Work out the finished part from the listing and answer in its coordinate system (mm). A direction names the side the tool comes from. Round coordinates to 2 decimals unless told otherwise and drop trailing zeros. Order: outer loops, then holes, each group sorted by start corner. A loop starts at its lowest first (then second) coordinate and runs counter-clockwise, first axis right, second up. Notation, with made-up numbers: (3, 3.5) - (8, 3.5) arc R31 cw to (8, 27.5) - close; hole circle Ø8 at (70, 70.25). An arc over 180 degrees is marked (long way). One line per question, with ' | ' between items. Start each with the question number.
from build123d import *

# Parameters (mm, degrees)
F1_DEPTH = 1285
F2_W     = 650
F2_H     = 250
F3_DEPTH = 650


with BuildPart() as f1:
    # F0 (on Front) → F1 (new body)
    with BuildSketch(Plane.XZ):
        Polygon((-600, 0), (0, 0), (600, 0), (600, 550), (550, 600), (-550, 600), (-600, 550), align=None)
    extrude(amount=F1_DEPTH)

    # F2 (on face) → F3 (cut)
    with BuildSketch(Plane.XZ.offset(1285)):
        with Locations((0, 125)):
            Rectangle(F2_W, F2_H)
    extrude(amount=-F3_DEPTH, mode=Mode.SUBTRACT)


solid = f1.part
1) Determine the mould class of faces 1 (the flat face through (-325, -965, 123)), 2 (the flat face through (-8, -491, 0)), 3 (the flat face through (-5, -965, 250)), 4 (the flat face through (-600, -634, 279)) for opening direction X: released by +X, released by -X, zero draft, split by the parting line, or undercut.
2) Section C-C on z = 46.5 is taken. Give the vertices of the cut face in (x, y).
3) For faces 5 (the flat face through (-575, -634, 575)), 6 (the flat face through (-5, -635, 127)), determine the directions among +Z, -Z, +X, -X, +Y, -Y from which every point of the face is accessible in a straight line to the end or side of a thin tool.
4) Section A-A on y = -795 is taken. Give the vertices of the cut face in (x, z), and give its area (3 significant figures).
5) Straight lines are drawn through the part: line 1 (Z direction, x = -2.5, y = -1100); line 2 (Y direction, x = -83, z = 40); line 3 (X direction, y = -958, z = 229). For each, find the intervals that lie inside material, in ascending order.
6) A flat-ended cylindrical pin translates along its axis: pin 1 (4 mm diameter, centred on x = 149, y = -849.5, fed in from -Z). Find the tip coordinate at first contact, or state that the pin passes through.
7) Section B-B on x = -163 is taken. Give the vertices of the cut face in (y, z).
Recorded:
1) face 1: undercut | face 2: zero draft | face 3: undercut | face 4: released by -X
2) outline: (-600, -1285) - (-325, -1285) - (-325, -635) - (325, -635) - (325, -1285) - (600, -1285) - (600, 0) - (-600, 0) - close
3) face 5: +Z, -X, +Y, -Y | face 6: -Z, -Y
4) outline: (-600, 0) - (-325, 0) - (-325, 250) - (325, 250) - (325, 0) - (600, 0) - (600, 550) - (550, 600) - (-550, 600) - (-600, 550) - close | area: 555,000 mm²
5) line 1: z = 250 to 600 | line 2: y = -635 to 0 | line 3: x = -600 to -325, 325 to 600
6) pin 1: stops at z = 250
7) outline: (-1285, 250) - (-635, 250) - (-635, 0) - (0, 0) - (0, 600) - (-1285, 600) - close
